Source: CAD feature listing. Evaluate the final solid. Frame: model axes, mm. A direction names the side the tool comes from. Give positions to 0.01 mm unless a question says otherwise; leave off trailing zeros. Loops run counter-clockwise (first coordinate to the right, second up) from the corner with the lowest first, then second, coordinate; pieces in that order, holes last.
Autodesk Inventor part; units mm, degrees
ref_plane "YZ Plane" through (0, 0, 0) normal (1, 0, 0) x (0, 1, 0)
ref_plane "XZ Plane" through (0, 0, 0) normal (0, 1, 0) x (-1, 0, 0)
ref_plane "XY Plane" through (0, 0, 0) normal (0, 0, 1) x (1, 0, 0)
sketch "Sketch1" plane through (0, 0, 0) normal (0, 0, 1) x (1, 0, 0)
  line L0 (0, 0) -> (42.2, 0)
  line L1 (42.2, 0) -> (42.2, 42.2)
  line L2 (42.2, 42.2) -> (0, 42.2)
  line L3 (0, 42.2) -> (0, 0)
  line L4 (0, 0) -> (5, 0)
  line L5 (42.2, 0) -> (45, 0)
  line L6 (5.6, 36.6) -> (36.6, 36.6) construction
  line L7 (36.6, 36.6) -> (36.6, 5.6) construction
  line L8 (36.6, 5.6) -> (5.6, 5.6) construction
  line L9 (5.6, 5.6) -> (5.6, 36.6) construction
  circle A0 centre (21.1, 21.1) radius 12
  line L10 (0.1, 42.1) -> (42.1, 42.1)
  line L11 (42.1, 42.1) -> (42.1, 0.1)
  line L12 (42.1, 0.1) -> (0.1, 0.1)
  line L13 (0.1, 0.1) -> (0.1, 42.1)
  line L14 (42.2, 42.2) -> (47.2, 42.2)
  line L15 (47.2, 42.2) -> (47.2, 21.1)
  line L16 (47.2, 21.1) -> (42.2, 21.1)
  line L17 (42.2, 21.1) -> (42.2, 42.2)
  line L18 (0, 42.2) -> (-5, 42.2)
  line L19 (-5, 42.2) -> (-5, 0)
  line L20 (-5, 0) -> (0, 0)
  line L21 (0, 0) -> (0, 42.2)
  point P0 (36.6, 21.1)
  point P1 (42.1, 21.1)
  point P2 (21.1, 36.6)
  point P3 (21.1, 42.1)
  point P4 (21.1, 42.2)
  dimension "d0" = 31
  dimension "d1" = 42
  dimension "d5" = 0.1
  dimension "d6" = 0.1
  dimension "d7" = 24
  dimension "d32" = 5
  dimension "d37" = 5
extrude "Extrusion2" add sketch "Sketch1" along normal blind 5 contours L3 L2 L1 L0 | L10 L11 L12 L13
extrude "Extrusion4" add sketch "Sketch1" along normal blind 44.6 contours L14 L15 L16 L1
extrude "Extrusion5" add sketch "Sketch1" along normal blind 24.6 contours L20 L19 L18 L3
hole "Hole1" at (5.6, 36.6, 0) at (36.6, 36.6, 0) at (36.6, 5.6, 0) at (5.6, 5.6, 0) direction (0, 0, 1) diameter 3.2 end through all
sketch "Sketch4" plane through (42.2, 42.2, 44.6) normal (0, 1, 0) x (1, 0, 0)
  line L0 (-47.2, 20) -> (-67.2, 20)
  line L1 (-67.2, 20) -> (-67.2, 25)
  line L2 (-67.2, 25) -> (-47.2, 25)
  line L3 (-47.2, 25) -> (-47.2, 20)
  point P0 (-42.2, 44.6)
  dimension "d42" = 20
  dimension "d43" = 5
extrude "Extrusion6" add sketch "Sketch4" against normal up to surface (42.2 mm away)
sketch "Sketch5" plane through (47.2, 21.1, 44.6) normal (1, 0, 0) x (0, 0, -1)
  line L0 (0, 0) -> (0, 21.1)
  line L1 (44.6, 21.1) -> (0, 21.1)
  line L2 (44.6, 0) -> (0, 0)
  point P0 (44.6, -21.1)
  point P1 (10, 10.55)
  point P2 (49.6, 26)
  point P3 (49.6, 0)
  dimension "d46" = 10
  dimension "d47" = 10.55
  dimension "d48" = 10.55
sketch "Sketch6" plane through (-5, 42.2, 19.6) normal (0, 0, -1) x (-1, 0, 0)
  line L0 (0, -42.2) -> (20, -42.2)
  line L1 (20, 0) -> (20, -42.2)
  line L2 (0, 0) -> (20, 0)
  line L3 (0, -42.2) -> (0, 0)
  point P0 (-5, -42.2)
  point P1 (10, -10)
  point P2 (10, -30)
  point P3 (10, -42.2)
  point P4 (10, 0)
  dimension "d49" = 10
  dimension "d65" = 20
hole "Hole3" at (-15, 32.2, 19.6) at (-15, 12.2, 19.6) direction (0, 0, 1) diameter 3.2 end through all
hole "Hole4" at (47.2, 31.65, 34.6) direction (-1, 0, 0) diameter 3.2 end through all
sketch "Sketch7" plane through (42.2, 0, 5) normal (1, 0, 0) x (0, 0, -1)
  line L0 (5, 21.1) -> (0, 21.1)
  line L1 (0, 0) -> (0, 21.1)
  line L2 (5, 0) -> (0, 0)
  line L3 (5, 0) -> (5, 21.1)
  point P0 (5, 0)
extrude "Extrusion7" add sketch "Sketch7" along normal blind 5
thicken "Thicken2" operation cut thickness 1 both sides no extend neighbours no toward (0, 1, 0) faces at (45.5333, 21.1, 18.2)
fillet "Fillet1" radius 2 8 edges at (0, 21.1, 24.6) (-25, 21.1, 24.6) (-25, 21.1, 19.6) (-5, 21.1, 19.6) (-5, 21.1, 0) (47.2, 21.1, 0) (42.2, 32.15, 44.6) (47.2, 32.15, 44.6)
equation "\"d6\" = d5"
properties part number "Motor Mount"
(1) First-contact query: pin 1 (17.5 mm diameter, centred on x = -15.5, y = 31, fed in from -Z); pin 2 (5 mm diameter, centred on x = 10.5, y = 28, fed in from +Z); pin 3 (23 mm diameter, centred on x = -14.5, y = 20, fed in from +Z). Flat tips, straight axial feed; report the tip coordinate or a pass-through.
A:
pin 1: stops at z = 19.58
pin 2: stops at z = 5
pin 3: stops at z = 24.6
(2) Mould query, pull axis X, two halves, no side actions, for faces 5 (the flat face through (45, 22.1, 25)), 6 (the cylindrical face through (46.6, 20.8, 0.57)), 7 (the flat face through (29, 11, 5)). Classes: pulls with the +X half, pulls with the -X half, needs draft (parallel to the pull), parting line crosses it, or undercut.
A:
face 5: needs draft
face 6: pulls with the +X half
face 7: undercut
(3) Section C-C, the plane z = 12. Return the cut outline in (x, y), then the cut area to 4 significant figures.
A:
outline: (-5, 0) - (0, 0) - (0, 42.2) - (-5, 42.2) - close; (42.2, 22.1) - (47.2, 22.1) - (47.2, 42.2) - (42.2, 42.2) - close
area: 311.5 mm2
(4) Ray query, line 1 along Y through (x, z) = (5.6, 3.1); line 2 along X through (y, z) = (5.6, 2.3); line 3 along Y through (x, z) = (36, 2). Return the intervals inside material, ascending.
A:
line 1: y = 0 to 4, 7.2 to 35, 38.2 to 42.2
line 2: x = -5 to 4, 7.2 to 35, 38.2 to 47.2
line 3: y = 0 to 4.12, 7.08 to 35.12, 38.08 to 42.2
(5) Reachability of faces 1 (the flat face through (-12, 21, 24.6)), 2 (the flat face through (-15, 21, 19.6)), 3 (the cylindrical face through (46.63, 32.01, 44)), 4 (the flat face through (42.2, 32, 24)) from +Z, -Z, +X, -X, +Y, -Y: full face, straight path, thin tool, end or side. Return the list, or none.
A:
face 1: +Z, -X, +Y, -Y
face 2: -Z, -X, +Y, -Y
face 3: +Z, +X, +Y, -Y
face 4: +Z, +Y, -Y
(6) Section B-B, the plane x = -15. Return the cut outline in (y, z).
A:
outline: (0, 19.6) - (10.6, 19.6) - (10.6, 24.6) - (0, 24.6) - close; (13.8, 19.6) - (30.6, 19.6) - (30.6, 24.6) - (13.8, 24.6) - close; (33.8, 19.6) - (42.2, 19.6) - (42.2, 24.6) - (33.8, 24.6) - close
(7) Section A-A, the plane y = 36.6. Return the cut outline in (x, z), then the cut area to 3 significant figures.
A:
outline: (-25, 21.6) arc R2 ccw to (-23, 19.6) - (-7, 19.6) arc R2 cw to (-5, 17.6) - (-5, 2) arc R2 ccw to (-3, 0) - (4, 0) - (4, 5) - (0, 5) - (0, 22.6) arc R2 ccw to (-2, 24.6) - (-23, 24.6) arc R2 ccw to (-25, 22.6) - close; (7.2, 0) - (35, 0) - (35, 5) - (7.2, 5) - close; (38.2, 0) - (45.2, 0) arc R2 ccw to (47.2, 2) - (47.2, 42.6) arc R2 ccw to (45.2, 44.6) - (44.2, 44.6) arc R2 ccw to (42.2, 42.6) - (42.2, 5) - (38.2, 5) - close
area: 620 mm2
(8) Section D-D, the plane y = 21.1. Return the cut outline in (x, z).
A:
outline: (-25, 21.6) arc R2 ccw to (-23, 19.6) - (-7, 19.6) arc R2 cw to (-5, 17.6) - (-5, 2) arc R2 ccw to (-3, 0) - (9.1, 0) - (9.1, 5) - (0, 5) - (0, 22.6) arc R2 ccw to (-2, 24.6) - (-23, 24.6) arc R2 ccw to (-25, 22.6) - close; (33.1, 0) - (45.2, 0) arc R2 ccw to (47.2, 2) - (47.2, 5) - (33.1, 5) - close
